Geometry check sheet. Reference: the model listing, model coordinates, mm. A direction names the side the tool comes from. Give positions to 0.01 mm unless a question says otherwise; leave off trailing zeros. Loops run counter-clockwise (first coordinate to the right, second up) from the corner with the lowest first, then second, coordinate; pieces in that order, holes last. Notation, with made-up numbers: (-16, 62) -> (30, 62) arc R9 ccw to (30, 79) -> close; hole circle Ø5 at (-13, -2). An arc over 180 degrees is marked (long way). One line per item, written item: value. Start each with the question number.
(1) Sectioned sample at C-C, the plane y = -42.5. Record the cut outline in (x, z), then the cut area to 3 significant figures.
(2) Draft check along Y on faces 3 (the face through (30, -80, 0)), 4 (the face through (30.07, -35.346, 2.253)), 5 (the face through (25, -50.3, -0.4)), 6 (the face through (-29.93, -35.346, 2.253)). Enter one of: pulls with the +Y half, pulls with the -Y half, needs draft (parallel to the pull), parting line crosses it, or undercut.
(3) Tool access check on faces 1 (the face through (-25, -50.3, -0.4)), 2 (the face through (0, 0, 14)). Record the directions out of +Z, -Z, +X, -X, +Y, -Y that give a thin tool (end or side, any length) a straight path to the whole face; none if there is none.
(4) Sectioned sample at B-B, the plane x = 0. Record the cut outline in (y, z), then the cut area to 3 significant figures.
(5) Scan lines: line 1 along X through (y, z) = (-31.5, -19); line 2 along Z through (x, y) = (0, -2); line 3 along Z through (x, y) = (-29, -42). Record each from-to range of solid material in increasing order. Write a range as from..to.
(6) Sectioned sample at A-A, the plane y = -27. Record the cut outline in (x, z).
(7) Gauge pin test, flat end, axial feed: pin 1 Ø12 at (x, z) = (-18, -5.5) entering from -Y. Record the tip position at first contact, or that the pin passes through.
(8) Sectioned sample at D-D, the plane z = 0. Record the cut outline in (x, y), then the cut area to 4 significant figures.
from build123d import *

# Parameters (mm, degrees)
F0_W     = 70
F0_H     = 60
F0_R     = 12.5
F1_DEPTH = 5
F2_W     = 10
F2_H     = 60
F3_DEPTH = 75
F4_R     = 7.5
F5_DEPTH = 70.001


with BuildPart() as f1:
    # F0 (on Front) → F1 (new body)
    with BuildSketch(Plane.XZ):
        Rectangle(F0_W, F0_H)
        Circle(F0_R, mode=Mode.SUBTRACT)
    extrude(amount=F1_DEPTH)

    # F2 (on face) → F3 (join)
    with BuildSketch(Plane.XZ.offset(5)):
        with Locations((-30, 0)):
            Rectangle(F2_W, F2_H)
        with Locations((30, 0)):
            Rectangle(F2_W, F2_H)
    extrude(amount=F3_DEPTH)

    # F4 (on face) → F5 (cut, through all)
    with BuildSketch(Plane.YZ.offset(35)):
        with Locations((-42.5, 0)):
            Circle(F4_R)
    extrude(amount=-F5_DEPTH, mode=Mode.SUBTRACT)


solid = f1.part
Calculated:
1. outline: (-35, -30) -> (-25, -30) -> (-25, -7.5) -> (-35, -7.5) -> close; (-35, 7.5) -> (-25, 7.5) -> (-25, 30) -> (-35, 30) -> close; (25, -30) -> (35, -30) -> (35, -7.5) -> (25, -7.5) -> close; (25, 7.5) -> (35, 7.5) -> (35, 30) -> (25, 30) -> close
1. area: 900 mm2
2. face 3: pulls with the -Y half
2. face 4: undercut
2. face 5: needs draft
2. face 6: undercut
3. face 1: +Z, -Z, -Y
3. face 2: +Z, -Z, +X, -X, +Y
4. outline: (-5, -30) -> (0, -30) -> (0, -12.5) -> (-5, -12.5) -> close; (-5, 12.5) -> (0, 12.5) -> (0, 30) -> (-5, 30) -> close
4. area: 175 mm2
5. line 1: x = -35..-25, 25..35
5. line 2: z = -30..-12.5, 12.5..30
5. line 3: z = -30..-7.48, 7.48..30
6. outline: (-35, -30) -> (-25, -30) -> (-25, 30) -> (-35, 30) -> close; (25, -30) -> (35, -30) -> (35, 30) -> (25, 30) -> close
7. pin 1: stops at y = -5
8. outline: (-35, -80) -> (-25, -80) -> (-25, -50) -> (-35, -50) -> close; (-35, -35) -> (-25, -35) -> (-25, -5) -> (-12.5, -5) -> (-12.5, 0) -> (-35, 0) -> close; (12.5, -5) -> (25, -5) -> (25, -35) -> (35, -35) -> (35, 0) -> (12.5, 0) -> close; (25, -80) -> (35, -80) -> (35, -50) -> (25, -50) -> close
8. area: 1,425 mm2
